Geometry: final body of the model. Coordinates: model frame, mm. A direction names the side the tool comes from. Coordinates: 2 decimals unless noted, no trailing zeros. Write each loop counter-clockwise with the first axis right and the second up, starting at its lowest first coordinate (ties: lowest second). Pieces come first, ordered by that corner, then holes. Notation, with made-up numbers: (25.5, 86) -> (71.5, 86) arc R25 cw to (71.5, 117) -> close; hole circle Ø4 at (-38.5, -37). An arc over 180 degrees is marked (long way). One line per item, written item: value.
```python
from build123d import *

# Parameters (mm, degrees)
F0_W     = 1905
F0_H     = 965.2
F1_DEPTH = 165.1
F2_T     = -2.54
F3_R     = 5.08


with BuildPart() as f1:
    # F0 (on Top) → F1 (new body)
    with BuildSketch(Plane.XY):
        Rectangle(F0_W, F0_H)
    extrude(amount=F1_DEPTH)

    # F2 (hollow: no face is removed)
    offset(amount=F2_T, mode=Mode.SUBTRACT)

    # F3
    f3_edges = [f1.edges().sort_by_distance(p)[0] for p in [
        (-952.5, -482.6, 82.55),
        (952.5, -482.6, 82.55),
        (0, -482.6, 0),
        (0, -482.6, 165.1),
        (-952.5, 482.6, 82.55),
        (-952.5, 0, 0),
        (-952.5, 0, 165.1),
        (952.5, 0, 165.1),
        (0, 482.6, 165.1),
        (952.5, 0, 0),
        (0, 482.6, 0),
        (952.5, 482.6, 82.55),
    ]]
    fillet(f3_edges, radius=F3_R)


solid = f1.part
```
(1) Line query: line 1 (Z direction, x = 333.5, y = 131); line 2 (Y direction, x = -685, z = 157); line 3 (X direction, y = 223.5, z = 138.5). Output: solid intervals per line, ascending. Write a range as [from, to].
Responses:
line 1: z = [0, 2.54], [162.56, 165.1]
line 2: y = [-482.6, -480.06], [480.06, 482.6]
line 3: x = [-952.5, -949.96], [949.96, 952.5]
(2) Pull-direction query (Y, two-part tool) for faces 3 (the flat face through (-13, 7, 0)), 4 (the flat face through (-13, -482.6, 81)), 5 (the flat face through (-13, 482.6, 81)), 6 (the flat face through (-13, 7, 162.56)); classes: released by +Y, released by -Y, zero draft, split by the parting line, or undercut.
Responses:
face 3: zero draft
face 4: released by -Y
face 5: released by +Y
face 6: undercut
(3) Section B-B (y = 72). Return the cut outline in (x, z), then the cut area to 3 significant figures.
Responses:
outline: (-952.5, 5.08) arc R5.08 ccw to (-947.42, 0) -> (947.42, 0) arc R5.08 ccw to (952.5, 5.08) -> (952.5, 160.02) arc R5.08 ccw to (947.42, 165.1) -> (-947.42, 165.1) arc R5.08 ccw to (-952.5, 160.02) -> close; hole (-949.96, 2.54) -> (949.96, 2.54) -> (949.96, 162.56) -> (-949.96, 162.56) -> close
area: 10,500 mm2
(4) Reachability of faces 1 (the flat face through (-13, 480.06, 81)), 2 (the flat face through (-13, 7, 165.1)) from +Z, -Z, +X, -X, +Y, -Y: full face, straight path, thin tool, end or side. Return the list, or none.
Responses:
face 1: none
face 2: +Z, +X, -X, +Y, -Y
(5) Section A-A (z = 142). Return the cut outline in (x, y), then the cut area to 3 significant figures.
Responses:
outline: (-952.5, -477.52) arc R5.08 ccw to (-947.42, -482.6) -> (947.42, -482.6) arc R5.08 ccw to (952.5, -477.52) -> (952.5, 477.52) arc R5.08 ccw to (947.42, 482.6) -> (-947.42, 482.6) arc R5.08 ccw to (-952.5, 477.52) -> close; hole (-949.96, -480.06) -> (949.96, -480.06) -> (949.96, 480.06) -> (-949.96, 480.06) -> close
area: 14,500 mm2
